Part model, mm, in its own coordinate system. Give positions to 0.01 mm unless a question says otherwise; leave off trailing zeros. Write each loop counter-clockwise with the first axis right and the second up, starting at its lowest first coordinate (ties: lowest second). Pieces come first, ordered by that corner, then holes.
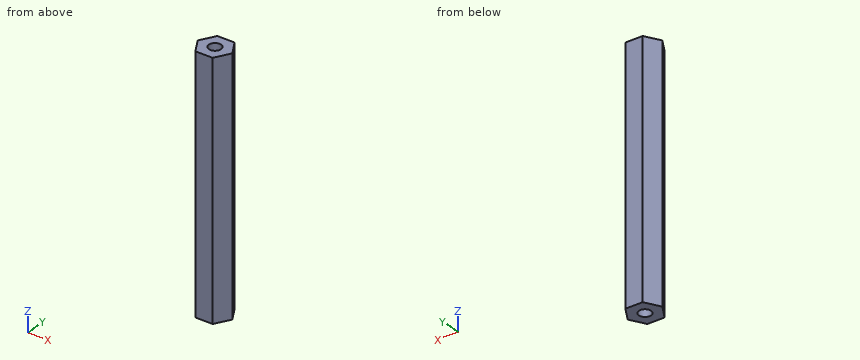
Autodesk Inventor part; units mm, degrees
ref_plane "Work Plane1" through (0, 0, 25) normal (0, 0, -1) x (-1, 0, 0)
ref_plane "YZ Plane" through (0, 0, 0) normal (1, 0, 0) x (0, 1, 0)
ref_plane "XZ Plane" through (0, 0, 0) normal (0, 1, 0) x (-1, 0, 0)
sketch "Sketch1" plane through (0, 0, 0) normal (0, 0, 1) x (1, 0, 0)
  line L0 (1.7321, 3) -> (3.4641, 0)
  line L1 (3.4641, 0) -> (1.7321, -3)
  line L2 (1.7321, -3) -> (-1.7321, -3)
  line L3 (-1.7321, -3) -> (-3.4641, 0)
  line L4 (-3.4641, 0) -> (-1.7321, 3)
  line L5 (-1.7321, 3) -> (1.7321, 3)
  point P0 (0, 0)
  point P1 (0, 0)
  dimension "d0" = 6
extrude "Extrusion1" add sketch "Sketch1" along normal blind 50
sketch "Sketch2" plane through (0, 0, 0) normal (0, 0, -1) x (-1, 0, 0)
  line L0 (-1.7321, 3) -> (1.7321, 3)
  line L1 (-3.4641, 0) -> (-1.7321, 3)
  line L2 (-1.7321, -3) -> (-3.4641, 0)
  line L3 (1.7321, -3) -> (-1.7321, -3)
  line L4 (3.4641, 0) -> (1.7321, -3)
  line L5 (1.7321, 3) -> (3.4641, 0)
  point P0 (0, 0)
  point P1 (0, 0)
hole "Hole1" at (0, 0, 0) direction (0, 0, 1) diameter 2.459 depth 7.5
ref_plane "Work Plane1" through (0, 0, 25) normal (0, 0, -1) x (-1, 0, 0)
mirror "Mirror1" about plane through (0, 0, 25) normal (0, 0, -1) of "Hole1"
properties part number "Wurth 970500361"
1) Saw through at C-C, the plane y = 2.3. Write the cut outline in (x, z).
Answers follow:
outline: (-2.14, 0) - (2.14, 0) - (2.14, 50) - (-2.14, 50) - close
2) Wall check: L1, parallel to X at y = 0, z = 6.25; L2, parallel to Y at x = 0, z = 4; L3, parallel to Y at x = -2.75, z = 39. Give the ranges that are in metal, low to high.
Answers follow:
L1: x = -3.46 to -1.23, 1.23 to 3.46
L2: y = -3 to -1.23, 1.23 to 3
L3: y = -1.24 to 1.24
3) Pin check, flat tips, straight feed: pin 1 Ø0.7 at (x, y) = (0, 0) entering from -Z; pin 2 Ø0.7 at (x, y) = (0.5, 0.5) entering from +Z; pin 3 Ø1 at (y, z) = (-1, 39) entering from -X. Stop position of each tip, or through.
Answers follow:
pin 1: stops at z = 7.5
pin 2: stops at z = 42.5
pin 3: stops at x = -3.18
4) Saw through at D-D, the plane y = -2.5. Write the cut outline in (x, z).
Answers follow:
outline: (-2.02, 0) - (2.02, 0) - (2.02, 50) - (-2.02, 50) - close
5) Saw through at A-A, the plane z = 43. Write the cut outline in (x, y), then the cut area to 3 significant figures.
Answers follow:
outline: (-3.46, 0) - (-1.73, -3) - (1.73, -3) - (3.46, 0) - (1.73, 3) - (-1.73, 3) - close; hole circle Ø2.46 at (0, 0)
area: 26.4 mm2
6) Saw through at B-B, the plane x = 0. Write the cut outline in (y, z), then the cut area to 3 significant figures.
Answers follow:
outline: (-3, 0) - (-1.23, 0) - (-1.23, 7.5) - (1.23, 7.5) - (1.23, 0) - (3, 0) - (3, 50) - (1.23, 50) - (1.23, 42.5) - (-1.23, 42.5) - (-1.23, 50) - (-3, 50) - close
area: 263 mm2
